from build123d import *

# Parameters (mm, degrees)
CROQUIS1_W              = 10
CROQUIS1_H              = 25
CROQUIS1_W_2            = 2.5
CROQUIS1_H_2            = 14.7771813
SALIENTE_EXTRUIR1_DEPTH = 2.5
REDONDEO1_R             = 2


with BuildPart() as part:
    # Croquis1 → Saliente-Extruir1 (new body)
    with BuildSketch(Plane.XY):
        Rectangle(CROQUIS1_W, CROQUIS1_H)
        Rectangle(CROQUIS1_W_2, CROQUIS1_H_2, mode=Mode.SUBTRACT)
    extrude(amount=SALIENTE_EXTRUIR1_DEPTH)

    # Redondeo1
    redondeo1_edges = [part.edges().sort_by_distance(p)[0] for p in [
        (5, -12.5, 1.25),
        (-5, -12.5, 1.25),
        (-5, 12.5, 1.25),
        (5, 12.5, 1.25),
    ]]
    fillet(redondeo1_edges, radius=REDONDEO1_R)


solid = part.part
Could you check a few things on this model? Use its own coordinates, in mm. A direction names the side the tool comes from. Give positions to 0.01 mm unless a question says otherwise; leave off trailing zeros. Write each loop counter-clockwise with the first axis right and the second up, starting at its lowest first coordinate (ties: lowest second). Pieces come first, ordered by that corner, then holes. Notation, with made-up numbers: (32.25, 82.25) - (65.25, 82.25) arc R28 cw to (65.25, 100.25) - close; hole circle Ø1 at (49, 36.5). An arc over 180 degrees is marked (long way). Use CSV: the item, a comma, the result in double quotes. Start each with the question number.
Item 1: I want a section at C-C, the plane z = 1.05. Please give me the cut outline in (x, y), then the cut area to 3 significant figures.
Item 2: I want a section at B-B, the plane x = -1. Please give me the cut outline in (y, z).
Item 3: If we mould it in two halves opening along Y, with no side actions, what happens to faces 3 (the face through (-5, 0, 1)), 4 (the face through (0, -7.389, 1)), 5 (the face through (-4.43, 11.9, 1.27)), 6 (the face through (4.4, -11.93, 1.27))? For each: pulls with the +Y half, pulls with the -Y half, needs draft (parallel to the pull), parting line crosses it, or undercut.
Item 4: For faces 1 (the face through (-1.25, 0, 1)), 2 (the face through (5, 0, 1)), which set-ups out of +Z, -Z, +X, -X, +Y, -Y let a thin tool reach every point of the face, with its end or its side?
Item 5: If I drill on line 1 along X through (y, z) = (1.25, 1.45); line 2 along Y through (x, z) = (-1, 1.55); line 3 along Y through (x, z) = (4.5, 0.1), over which ranges is the centre line in solid material (lowest first)?
Item 6: I want a section at A-A, the plane y = -6. Please give me the cut outline in (x, z).
Item 7: I'm going to push a flat-ended pin straight in: pin 1 (2 mm diameter, centred on x = 0, y = 4, fed in from -Z). Where does the tip first touch, or does it pass through?
Findings:
1,outline,"(-5, -10.5) arc R2 ccw to (-3, -12.5) - (3, -12.5) arc R2 ccw to (5, -10.5) - (5, 10.5) arc R2 ccw to (3, 12.5) - (-3, 12.5) arc R2 ccw to (-5, 10.5) - close; hole (-1.25, -7.39) - (1.25, -7.39) - (1.25, 7.39) - (-1.25, 7.39) - close"
1,area,"210 mm2"
2,outline,"(-12.5, 0) - (-7.39, 0) - (-7.39, 2.5) - (-12.5, 2.5) - close; (7.39, 0) - (12.5, 0) - (12.5, 2.5) - (7.39, 2.5) - close"
3,face 3,"needs draft"
3,face 4,"undercut"
3,face 5,"pulls with the +Y half"
3,face 6,"pulls with the -Y half"
4,face 1,"+Z, -Z"
4,face 2,"+Z, -Z, +X, +Y, -Y"
5,line 1,"x = -5 to -1.25, 1.25 to 5"
5,line 2,"y = -12.5 to -7.39, 7.39 to 12.5"
5,line 3,"y = -11.82 to 11.82"
6,outline,"(-5, 0) - (-1.25, 0) - (-1.25, 2.5) - (-5, 2.5) - close; (1.25, 0) - (5, 0) - (5, 2.5) - (1.25, 2.5) - close"
7,pin 1,"passes through"
